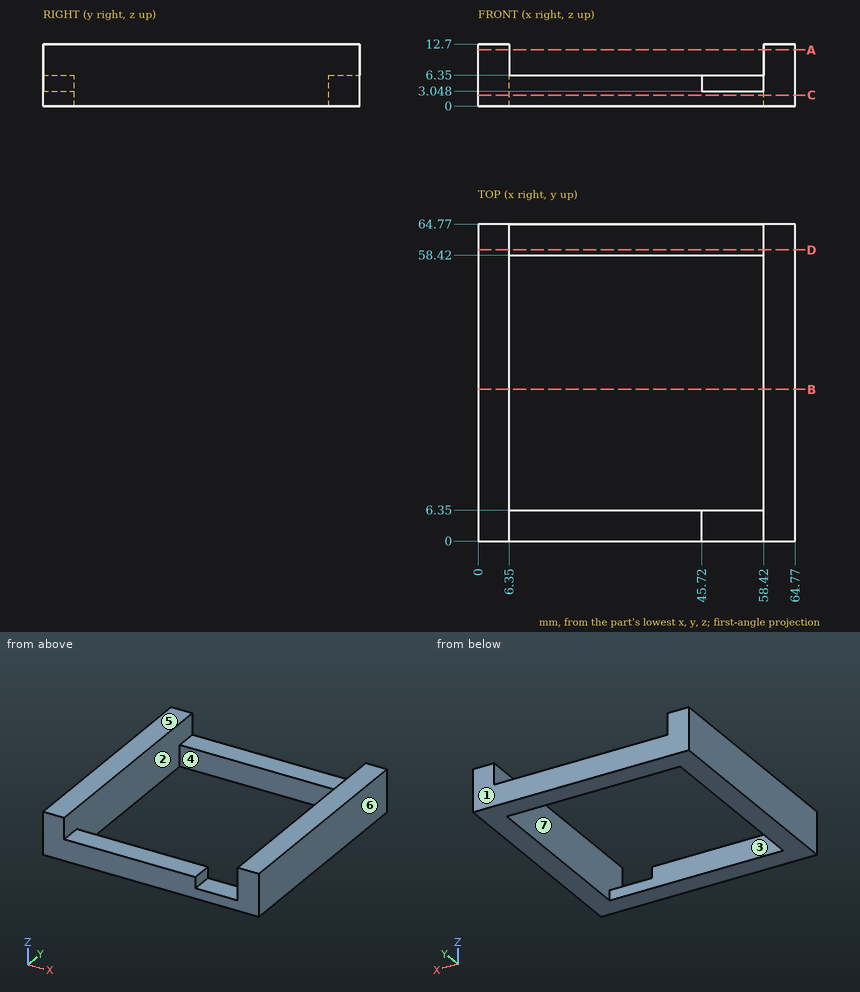
Here's the drawing with two shaded views (mm, measured from the low corner). I have some questions. A direction names the side the tool comes from. Coordinates: 2 decimals unless noted, no trailing zeros. Loops run counter-clockwise (first coordinate to the right, second up) from the corner with the lowest first, then second, coordinate; pieces in that order, holes last.
Item 1: Which directions (+Z, -Z, +X, -X, +Y, -Y) give clear straight access to the entire face, cutting with the end or side of a thin tool? Please do the marked faces 1, 2 and 3.
Answers below:
face 1: +Z, -Z, +X, -X, +Y
face 2: +Z
face 3: +Z, -Z
Item 2: If we mould it in two halves opening along X, with no side actions, what happens to the marked faces 4, 5, 6 and 7? For each: released by +X, released by -X, zero draft, split by the parting line, or undercut.
Answers below:
face 4: undercut
face 5: zero draft
face 6: released by +X
face 7: undercut
Item 3: I'm going to push flat-ended pins straight in: pin 1 (3 mm diameter, centred on x = 35, y = 63, fed in from +Z); pin 2 (7 mm diameter, centred on x = 53.5, y = 2.5, fed in from +Z). Where does each tip first touch, or does it pass through?
Answers below:
pin 1: stops at z = 6.35
pin 2: stops at z = 3.05
Item 4: Suppose I cut it at D-D (y = 59.5). Please give me the cut outline in (x, z), then the cut area to 3 significant figures.
Answers below:
outline: (0, 0) - (64.77, 0) - (64.77, 12.7) - (58.42, 12.7) - (58.42, 6.35) - (6.35, 6.35) - (6.35, 12.7) - (0, 12.7) - close
area: 492 mm2
Item 5: Please list where these lines run through material, in increasing order: L1, parallel to X at y = 8, z = 3.5; L2, parallel to Z at x = 48, y = 5.5.
Answers below:
L1: x = 0 to 6.35, 58.42 to 64.77
L2: z = 0 to 3.05
Item 6: Suppose I cut it at A-A (z = 11.5). Please give me the cut outline in (x, y).
Answers below:
outline: (0, 0) - (6.35, 0) - (6.35, 64.77) - (0, 64.77) - close; (58.42, 0) - (64.77, 0) - (64.77, 64.77) - (58.42, 64.77) - close
Item 7: Suppose I cut it at B-B (y = 31). Please give me the cut outline in (x, z), then the cut area to 3 significant figures.
Answers below:
outline: (0, 0) - (6.35, 0) - (6.35, 12.7) - (0, 12.7) - close; (58.42, 0) - (64.77, 0) - (64.77, 12.7) - (58.42, 12.7) - close
area: 161 mm2
Item 8: Suppose I cut it at C-C (z = 2.25). Please give me the cut outline in (x, y), then the cut area to 3 significant figures.
Answers below:
outline: (0, 0) - (64.77, 0) - (64.77, 64.77) - (0, 64.77) - close; hole (6.35, 6.35) - (58.42, 6.35) - (58.42, 58.42) - (6.35, 58.42) - close
area: 1,480 mm2
